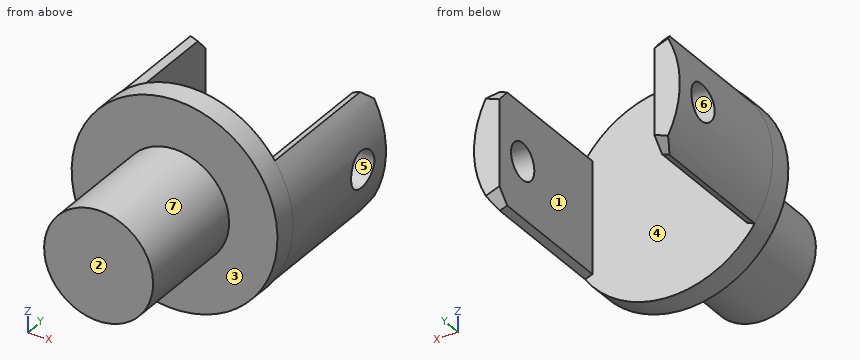
```python
from build123d import *

# Parameters (mm, degrees)
SKETCH1_R           = 42.5
BOSS_EXTRUDE1_DEPTH = 10
BOSS_EXTRUDE2_DEPTH = 60
SKETCH3_R           = 7.5
CUT_EXTRUDE1_DEPTH  = 111.709078219
SKETCH4_R           = 22.5
BOSS_EXTRUDE3_DEPTH = 49
CHAMFER1_SIZE       = 5
CHAMFER2_SIZE       = 5


with BuildPart() as part:
    # Sketch1 → Boss-Extrude1 (new body)
    with BuildSketch(Plane(origin=(0, 0, 0), x_dir=(1, 0, 0), z_dir=(0, 1, 0))):
        with Locations(Location((0, 0, 0), (0, 0, 270))):
            Circle(SKETCH1_R)
    extrude(amount=BOSS_EXTRUDE1_DEPTH)

    # Sketch2 → Boss-Extrude2 (add)
    with BuildSketch(Plane(origin=(0, 10, 0), x_dir=(1, 0, 0), z_dir=(0, 1, 0))):
        with BuildLine():
            Line((32, 27.968732542), (32, -27.968732542))
            ThreePointArc((32, -27.968732542), (42.5, 0), (32, 27.968732542))
        make_face()
    boss_extrude2 = extrude(amount=BOSS_EXTRUDE2_DEPTH)

    # Sketch3 → Cut-Extrude1 (cut, through all)
    with BuildSketch(Plane.ZY.offset(-32)):
        with Locations((0, 55)):
            Circle(SKETCH3_R)
    cut_extrude1 = extrude(amount=-CUT_EXTRUDE1_DEPTH, mode=Mode.SUBTRACT)

    # Mirror1: Boss-Extrude2, Cut-Extrude1 across plane
    add(boss_extrude2.mirror(Plane(origin=(0, 0, 0), x_dir=(0, 0, 1), z_dir=(1, 0, 0))))
    add(cut_extrude1.mirror(Plane(origin=(0, 0, 0), x_dir=(0, 0, 1), z_dir=(1, 0, 0))), mode=Mode.SUBTRACT)

    # Sketch4 → Boss-Extrude3 (add)
    with BuildSketch(Plane.XZ):
        with Locations(Location((0, 0, 0), (0, 0, 90))):
            Circle(SKETCH4_R)
    extrude(amount=BOSS_EXTRUDE3_DEPTH)

    # Chamfer1
    # the kernel refuses this chamfer: 5 mm, written as the material it takes off along each edge
    with BuildSketch(Plane(origin=(32, 10, -27.968732542), x_dir=(0.613569743675552, 0, 0.7896405319168447), z_dir=(0, 1, 0)), Plane(origin=(-32, 10, 27.968732542), x_dir=(-0.613569743675558, 0, -0.78964053191684), z_dir=(0, 1, 0))) as chamfer1_piece_1:
        with BuildLine():
            Line((4.902026088, 0), (CHAMFER1_SIZE * 0.789640531917, -CHAMFER1_SIZE * 0.613569743676))
            Line((CHAMFER1_SIZE * 0.789640531917, -CHAMFER1_SIZE * 0.613569743676), (0, 0))
            ThreePointArc((0, 0), (2.480684858, 0.070724564), (4.902026088, 0))
        make_face()
    extrude(amount=72.684374005, mode=Mode.SUBTRACT)
    with BuildSketch(Plane(origin=(32, 10, 27.968732542), x_dir=(0.6135697436755528, 0, -0.7896405319168441), z_dir=(0, 1, 0)), Plane(origin=(-32, 10, -27.968732542), x_dir=(-0.6135697436755566, 0, 0.7896405319168412), z_dir=(0, 1, 0))) as chamfer1_piece_2:
        with BuildLine():
            Line((4.902026088, 0), (CHAMFER1_SIZE * 0.789640531917, CHAMFER1_SIZE * 0.613569743676))
            Line((CHAMFER1_SIZE * 0.789640531917, CHAMFER1_SIZE * 0.613569743676), (0, 0))
            ThreePointArc((0, 0), (2.480684858, -0.070724564), (4.902026088, 0))
        make_face()
    extrude(amount=72.684374005, mode=Mode.SUBTRACT)

    # Chamfer2
    chamfer2_edges = [part.edges().sort_by_distance(p)[0] for p in [
        (33.503867445, 70, -23.533313298),
        (33.503867445, 70, 23.533313298),
        (-33.503867445, 70, 23.533313298),
        (-33.503867445, 70, -23.533313298),
    ]]
    chamfer(chamfer2_edges, length=CHAMFER2_SIZE)


solid = part.part
```
Work out the finished part from the listing and answer in its coordinate system (mm). Face numbers are marked on the shaded views. A direction names the side the tool comes from. Round coordinates to 2 decimals unless told otherwise and drop trailing zeros. Write each loop counter-clockwise with the first axis right and the second up, starting at its lowest first coordinate (ties: lowest second). Pieces come first, ordered by that corner, then holes. Notation, with made-up numbers: (50, 33.5) -> (63, 33.5) arc R11 ccw to (63, 40.5) -> close; hole circle Ø3 at (64, 74). An arc over 180 degrees is marked (long way). Write each question's results on one line, items separated by ' | '.
Q1. Straight lines are drawn through the part: line 1 along X through (y, z) = (41, -1); line 2 along Z through (x, y) = (35, 55) (3 decimals); line 3 along Y through (x, z) = (-40, 0). For each, find the intervals that lie inside material, in ascending order. Write a range as [from, to].
Data:
line 1: [-42.49, -32], [32, 42.49] | line 2: [-24.095, -7.5], [7.5, 24.095] | line 3: [0, 47.5], [62.5, 70]
Q2. Section C-C, the plane x = 0 is taken. Write down the section's boundary in (y, z).
Data:
outline: (-49, -22.5) -> (0, -22.5) -> (0, -42.5) -> (10, -42.5) -> (10, 42.5) -> (0, 42.5) -> (0, 22.5) -> (-49, 22.5) -> close
Q3. Section D-D, the plane y = 55 is taken. Write down the section's boundary in (x, z), then the cut area to 3 significant figures.
Data:
outline: (-41.83, -7.5) arc R42.5 ccw to (-35.01, -24.1) -> (-32, -22.97) -> (-32, -7.5) -> close; (-41.83, 7.5) -> (-32, 7.5) -> (-32, 22.97) -> (-35.01, 24.1) arc R42.5 ccw to start; (32, -22.97) -> (35.01, -24.1) arc R42.5 ccw to (41.83, -7.5) -> (32, -7.5) -> close; (32, 7.5) -> (41.83, 7.5) arc R42.5 ccw to (35.01, 24.1) -> (32, 22.97) -> close | area: 465 mm^2
Q4. Section A-A, the plane z = 0 is taken. Write down the section's boundary in (x, y), then the cut area to 3 significant figures.
Data:
outline: (-42.5, 0) -> (-22.5, 0) -> (-22.5, -49) -> (22.5, -49) -> (22.5, 0) -> (42.5, 0) -> (42.5, 47.5) -> (32, 47.5) -> (32, 10) -> (-32, 10) -> (-32, 47.5) -> (-42.5, 47.5) -> close; (-42.5, 62.5) -> (-32, 62.5) -> (-32, 70) -> (-42.5, 70) -> close; (32, 62.5) -> (42.5, 62.5) -> (42.5, 70) -> (32, 70) -> close | area: 4,000 mm^2
Q5. Which of the six approach directions +Z, -Z, +X, -X, +Y, -Y give full straight-line access (tool end or side, diameter ignored) to the marked faces 1, 2 and 3?
Data:
face 1: +Z, -Z, +Y | face 2: +Z, -Z, +X, -X, -Y | face 3: -Y
Q6. Determine the mould class of the marked faces 4, 5, 6 and 7 for opening direction Y: released by +Y, released by -Y, zero draft, split by the parting line, or undercut.
Data:
face 4: released by +Y | face 5: undercut | face 6: undercut | face 7: zero draft
Q7. Section B-B, the plane y = 32.5 is taken. Write down the section's boundary in (x, z).
Data:
outline: (-35.01, -24.1) -> (-32, -22.97) -> (-32, 22.97) -> (-35.01, 24.1) arc R42.5 ccw to start; (32, -22.97) -> (35.01, -24.1) arc R42.5 ccw to (35.01, 24.1) -> (32, 22.97) -> close
Q8. Flat-ended cylindrical pins translate along their axes: P1, Ø1, axis at x = -2.5, y = -4, coming from the +Z side; P2, Ø3, axis at y = 42, z = 8, coming from the -X side; P3, Ø12, axis at x = 17, z = 5.5, coming from the +Y side. Find the tip coordinate at first contact, or state that the pin passes through.
Data:
P1: z = 22.41 | P2: x = -42 | P3: y = 10
